Input: part model. Units: mm. Frame: model coordinates. A direction names the side the tool comes from. Coordinates: 2 decimals unless noted, no trailing zeros. Write each loop counter-clockwise with the first axis right and the second up, starting at its lowest first coordinate (ties: lowest second). Pieces come first, ordered by that corner, then holes.
1) Section query B-B (y = -7). Output: boundary loops of the cut face in (x, z) (3 decimals).
2) Line query: L1, parallel to Z at x = 0, y = -7 (3 decimals); L2, parallel to Z at x = 2.75, y = -2.25 (3 decimals); L3, parallel to Z at x = 0, y = -1 (3 decimals). Output: solid intervals per line, ascending.
3) Pin query (flat end, axial travel): pin 1 Ø4 at (x, z) = (1, -3) entering from +Y; pin 2 Ø6 at (y, z) = (-6.5, -2.5) entering from +X; pin 3 Ø4 at (x, z) = (-2, 5.5) entering from -Y; pin 4 Ø1.5 at (y, z) = (-6.5, 0) entering from -X. Return the tip coordinate at first contact, or that it passes through.
4) Section query A-A (x = 0). Output: boundary loops of the cut face in (y, z) (3 decimals), then the cut area to 3 significant figures.
5) Section query D-D (y = 2.5). Output: boundary loops of the cut face in (x, z) (1 decimal).
6) Set-up query: faces 3 (the flat face through (0, -8, 8)), 4 (the cylindrical face through (-0.108, -0.488, -4.039)), 5 (the cylindrical face through (0.23, -5.54, 7.58)). Return all of +Z, -Z, +X, -X, +Y, -Y with unobstructed straight access to the full face (end or side cutting, diameter ignored); none if empty.
7) Draft query along Z for faces 1 (the cylindrical face through (-0.108, -0.488, 4.039)), 2 (the flat face through (0, -8, -8)). Return one class per face: pulls with the +Z half, pulls with the -Z half, needs draft (parallel to the pull), parting line crosses it, or undercut.
8) Section query C-C (z = -4.5). Output: boundary loops of the cut face in (x, y).
from build123d import *

# Parameters (mm, degrees)
SKETCH1_R           = 4
BOSS_EXTRUDE1_DEPTH = 3.025
SKETCH3_R           = 0.5


with BuildPart() as part:
    # Sketch1 → Boss-Extrude1 (new, symmetric)
    with BuildSketch(Plane.XY):
        Circle(SKETCH1_R)
    extrude(amount=BOSS_EXTRUDE1_DEPTH, both=True)

    # Sweep1: sweep along a path in Sketch2
    with BuildLine(Plane(origin=(0, 0, 0), x_dir=(0, 0, -1), z_dir=(1, 0, 0))) as sweep1_path:
        Line((-3.025, 0), (-5.025, 0))
        ThreePointArc((-5.025, 0), (-7.146320344, -0.878679656), (-8.025, -3))
        Line((-8.025, -3), (-8.025, -8))
    # Sketch3 → Sweep1 (sweep)
    with BuildSketch(Plane.XY.offset(3.025)):
        Circle(SKETCH3_R)
    sweep1 = sweep(path=sweep1_path.line)

    # Mirror1: Sweep1 across plane
    add(sweep1.mirror(Plane.XY))


solid = part.part
Answer:
1. outline: circle Ø1 at (0, -8.025); circle Ø1 at (0, 8.025)
2. L1: z = -8.525 to -7.525, 7.525 to 8.525
2. L2: z = -3.025 to 3.025
2. L3: z = -7.897 to -6.525, -3.025 to 3.025, 6.525 to 7.897
3. pin 1: stops at y = 4
3. pin 2: stops at x = 1.94
3. pin 3: stops at y = -0.9
3. pin 4: passes through
4. outline: (-8, -8.525) - (-3, -8.525) arc R3.5 ccw to (0.5, -5.025) - (0.5, -3.025) - (4, -3.025) - (4, 3.025) - (0.5, 3.025) - (0.5, 5.025) arc R3.5 ccw to (-3, 8.525) - (-8, 8.525) - (-8, 7.525) - (-3, 7.525) arc R2.5 cw to (-0.5, 5.025) - (-0.5, 3.025) - (-4, 3.025) - (-4, -3.025) - (-0.5, -3.025) - (-0.5, -5.025) arc R2.5 cw to (-3, -7.525) - (-8, -7.525) - close
4. area: 71.8 mm2
5. outline: (-3.1, -3) - (3.1, -3) - (3.1, 3) - (-3.1, 3) - close
6. face 3: +Z, -Z, +X, -X, -Y
6. face 4: none
6. face 5: -Y
7. face 1: undercut
7. face 2: needs draft
8. outline: circle Ø1 at (0, 0)
